Source: CAD feature listing. Evaluate the final solid. Frame: model axes, mm. Face numbers are marked on the shaded views. A direction names the side the tool comes from. Give positions to 0.01 mm unless a question says otherwise; leave off trailing zeros. Order: outer loops, then holes, each group sorted by start corner. A loop starts at its lowest first (then second) coordinate and runs counter-clockwise, first axis right, second up.
1) Section C-C, the plane z = 2.5. Return loops of the section in (x, y), plus the area to 3 significant figures.
2) Section B-B, the plane x = -8.25. Return loops of the section in (y, z), plus the area to 3 significant figures.
3) Draft query along X for the marked faces 3, 4, 5 and 6. Return one class per face: released by +X, released by -X, zero draft, split by the parting line, or undercut.
4) First-contact query: P1, Ø8, axis at x = -4.5, z = 4, coming from the +Y side; P2, Ø3, axis at x = -1.5, z = 0.5, coming from the -Y side. Flat tips, straight axial feed; report the tip coordinate or a pass-through.
5) Material intervals for line 1 (Z direction, x = 5.5, y = 1.2); line 2 (X direction, y = 3.65, z = -8.5), sorted ascending.
6) Access query for the marked faces 1 and 2. Directions: +Z, -Z, +X, -X, +Y, -Y. A direction counts if a zero-diameter tool reaches every point of the face in a straight line with its end or side. Return the directions, or none.
7) Section A-A, the plane y = 1.45. Return loops of the section in (x, z).
```python
from build123d import *

# Parameters (mm, degrees)
SKETCH1_W           = 26
SKETCH1_H           = 26
SKETCH1_W_2         = 24
SKETCH1_H_2         = 24
BOSS_EXTRUDE1_DEPTH = 1
SKETCH1_3_W         = 24
SKETCH1_3_H         = 24
BOSS_EXTRUDE2_DEPTH = 2
SKETCH1_4_W         = 28
SKETCH1_4_H         = 28
SKETCH1_4_W_2       = 26
SKETCH1_4_H_2       = 26
BOSS_EXTRUDE3_DEPTH = 4
FILLET1_R           = 1
FILLET2_R           = 2


with BuildPart() as part:
    # Sketch1 → Boss-Extrude1 (new body)
    with BuildSketch(Plane(origin=(0, 0, 0), x_dir=(1, 0, 0), z_dir=(0, 1, 0))):
        Rectangle(SKETCH1_W, SKETCH1_H)
        Rectangle(SKETCH1_W_2, SKETCH1_H_2, mode=Mode.SUBTRACT)
    extrude(amount=BOSS_EXTRUDE1_DEPTH)

    # Sketch1<3> → Boss-Extrude2 (add)
    with BuildSketch(Plane(origin=(0, 0, 0), x_dir=(1, 0, 0), z_dir=(0, 1, 0))):
        Rectangle(SKETCH1_3_W, SKETCH1_3_H)
    extrude(amount=BOSS_EXTRUDE2_DEPTH)

    # Sketch1<4> → Boss-Extrude3 (add)
    with BuildSketch(Plane(origin=(0, 0, 0), x_dir=(1, 0, 0), z_dir=(0, 1, 0))):
        Rectangle(SKETCH1_4_W, SKETCH1_4_H)
        Rectangle(SKETCH1_4_W_2, SKETCH1_4_H_2, mode=Mode.SUBTRACT)
    extrude(amount=BOSS_EXTRUDE3_DEPTH)

    # Fillet1
    fillet1_edges = [part.edges().sort_by_distance(p)[0] for p in [
        (-12, 1.5, 12),
        (12, 1.5, 12),
        (12, 1.5, -12),
        (-12, 1.5, -12),
    ]]
    fillet(fillet1_edges, radius=FILLET1_R)

    # Fillet2
    fillet2_edges = [part.edges().sort_by_distance(p)[0] for p in [
        (13, 2.5, -13),
        (13, 2.5, 13),
        (-13, 2.5, 13),
        (-13, 2.5, -13),
    ]]
    fillet(fillet2_edges, radius=FILLET2_R)


solid = part.part
```
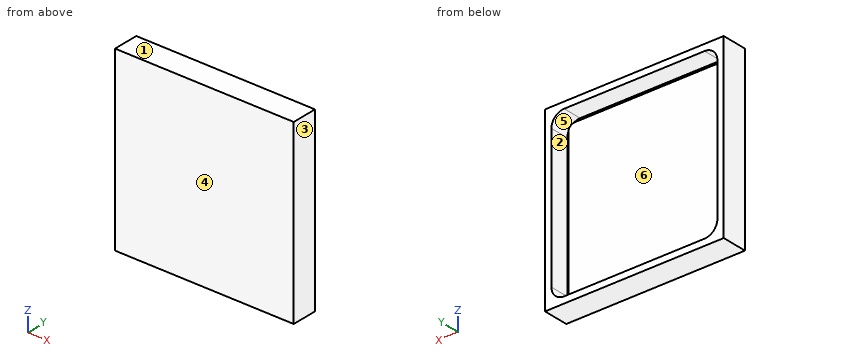
From the geometry:
1. outline: (-14, 0) - (14, 0) - (14, 4) - (13, 4) - (13, 1) - (12, 1) - (12, 2) - (-12, 2) - (-12, 1) - (-13, 1) - (-13, 4) - (-14, 4) - close
1. area: 58.0 mm2
2. outline: (0, -14) - (4, -14) - (4, -13) - (1, -13) - (1, -12) - (2, -12) - (2, 12) - (1, 12) - (1, 13) - (4, 13) - (4, 14) - (0, 14) - close
2. area: 58.0 mm2
3. face 3: released by +X
3. face 4: zero draft
3. face 5: undercut
3. face 6: undercut
4. P1: stops at y = 2
4. P2: stops at y = 0
5. line 1: z = -14 to -13, -12 to 12, 13 to 14
5. line 2: x = -14 to -13, 13 to 14
6. face 1: +Z, +X, -X, +Y, -Y
6. face 2: +Y
7. outline: (-14, -14) - (14, -14) - (14, 14) - (-14, 14) - close; (-12, -11) arc R1 ccw to (-11, -12) - (11, -12) arc R1 ccw to (12, -11) - (12, 11) arc R1 ccw to (11, 12) - (-11, 12) arc R1 ccw to (-12, 11) - close; hole (-13, -11) arc R2 ccw to (-11, -13) - (11, -13) arc R2 ccw to (13, -11) - (13, 11) arc R2 ccw to (11, 13) - (-11, 13) arc R2 ccw to (-13, 11) - close
